The listing builds one solid part. Answer for the finished solid, in the listing's coordinates (mm). Face numbers are marked on the shaded views. A direction names the side the tool comes from. Coordinates: 2 decimals unless noted, no trailing zeros. Order: outer loops, then holes, each group sorted by start corner. A loop starts at its lowest first (then second) coordinate and runs counter-clockwise, first axis right, second up. Notation, with made-up numbers: (58, 53.25) - (76, 53.25) arc R20 cw to (76, 79.25) - close; hole circle Ø4 at (-35, -15.5). An arc over 180 degrees is marked (long way). Use a Markdown table: item, result. Add a question column.
Item 1: Flat-ended cylindrical pins translate along their axes: P1, Ø2, axis at x = 4, y = 0.5, coming from the +Z side; P2, Ø3, axis at x = 5, y = 2.5, coming from the -Z side; P3, Ø0.6, axis at x = 2.5, z = 3, coming from the +Y side; P4, Ø2, axis at x = 2, y = 4, coming from the +Z side. Find the tip coordinate at first contact, or state that the pin passes through.
Item 2: The part is cut by section A-A, the plane y = 1.6. Give the vertices of the cut face in (x, z).
Item 3: The part is cut by section D-D, the plane z = 3.4. Give the vertices of the cut face in (x, y), then the cut area to 3 significant figures.
Item 4: The part is cut by section B-B, the plane z = 1.45. Give the vertices of the cut face in (x, y), then the cut area to 3 significant figures.
Item 5: For the marked faces 1 and 2, determine the directions among +Z, -Z, +X, -X, +Y, -Y from which every point of the face is accessible in a straight line to the end or side of a thin tool.
Item 6: The part is cut by section C-C, the plane x = 4.7. Give the vertices of the cut face in (y, z), then the cut area to 3 significant figures.
Item 7: Find the intervals of material crossed by line 1 along Z through (x, y) = (1.9, 3.1); line 2 along X through (y, z) = (0.35, 1.8) (3 decimals), in increasing order.
from build123d import *

# Parameters (mm, degrees)
SKETCH1_W           = 6
SKETCH1_H           = 5
BOSS_EXTRUDE1_DEPTH = 2
SKETCH2_W           = 6
SKETCH2_H           = 2
BOSS_EXTRUDE2_DEPTH = 2
CUT_EXTRUDE1_DEPTH  = 10
CUT_EXTRUDE2_DEPTH  = 10
CUT_EXTRUDE3_DEPTH  = 10


with BuildPart() as part:
    # Sketch1 → Boss-Extrude1 (new body)
    with BuildSketch(Plane.XY):
        with Locations((3, 2.5)):
            Rectangle(SKETCH1_W, SKETCH1_H)
    extrude(amount=BOSS_EXTRUDE1_DEPTH)

    # Sketch2 → Boss-Extrude2 (add)
    with BuildSketch(Plane.XY.offset(2)):
        with Locations((3, 1)):
            Rectangle(SKETCH2_W, SKETCH2_H)
    extrude(amount=BOSS_EXTRUDE2_DEPTH)

    # 3DSketch1 → Cut-Extrude1 (cut, along a direction that is not the sketch's normal)
    with BuildSketch(Plane(origin=(6, 0, 2), x_dir=(-0.816496580927726, 0.4082482904638629, 0.40824829046386285), z_dir=(-0.5345224838248487, -0.26726124191242434, -0.8017837257372732))):
        Polygon((0, 0), (3.265986324, -1.527525232), (4.898979486, 0), (1.632993162, 1.527525232), align=None)
    extrude(amount=-CUT_EXTRUDE1_DEPTH, dir=(-1, 0, 0), mode=Mode.SUBTRACT)

    # Sketch3 → Cut-Extrude2 (cut)
    with BuildSketch(Plane.XY.offset(2)):
        Polygon((6, 0), (5, 2), (3.5, 5), (6, 5), align=None)
    extrude(amount=-CUT_EXTRUDE2_DEPTH, mode=Mode.SUBTRACT)

    # Sketch4 → Cut-Extrude3 (cut)
    with BuildSketch(Plane.XY.offset(2)):
        with BuildLine():
            ThreePointArc((0, 2.084019689), (0.721936041, 3.994383965), (2.499411695, 5))
            Line((2.499411695, 5), (0, 5))
            Line((0, 5), (0, 2.084019689))
        make_face()
    extrude(amount=-CUT_EXTRUDE3_DEPTH, mode=Mode.SUBTRACT)


solid = part.part
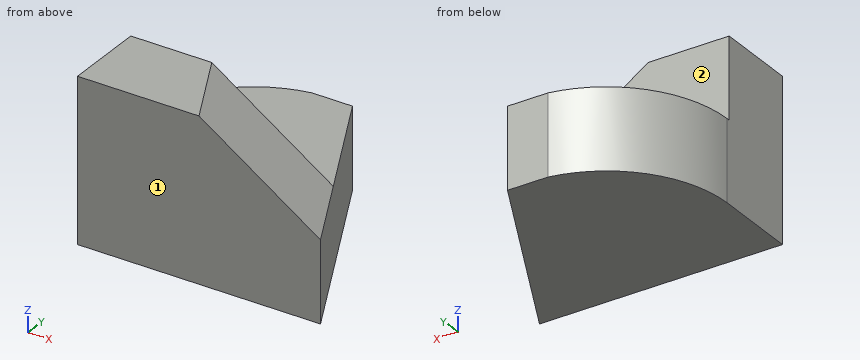
Solution:
| question | item | result |
|---|---|---|
| 1 | P1 | stops at z = 3.91 |
| 1 | P2 | stops at z = 0 |
| 1 | P3 | stops at y = 2 |
| 1 | P4 | stops at z = 2 |
| 2 | outline | (0, 0) - (5.2, 0) - (5.2, 2) - (2.2, 4) - (0, 4) - close |
| 3 | outline | (0, 0) - (3.9, 0) - (2.9, 2) - (0, 2) - close |
| 3 | area | 6.80 mm2 |
| 4 | outline | (0, 0) - (6, 0) - (3.5, 5) - (2.5, 5) arc R3 ccw to (0, 2.08) - close |
| 4 | area | 21.9 mm2 |
| 5 | face 1 | +Z, -Z, +X, -X, -Y |
| 5 | face 2 | +Z, +X, -X, +Y |
| 6 | outline | (0, 0) - (2.6, 0) - (2.6, 2) - (2, 2) - (2, 2.2) - (0, 2.87) - close |
| 6 | area | 6.27 mm2 |
| 7 | line 1 | z = 0 to 2 |
| 7 | line 2 | x = 0 to 5.825 |
